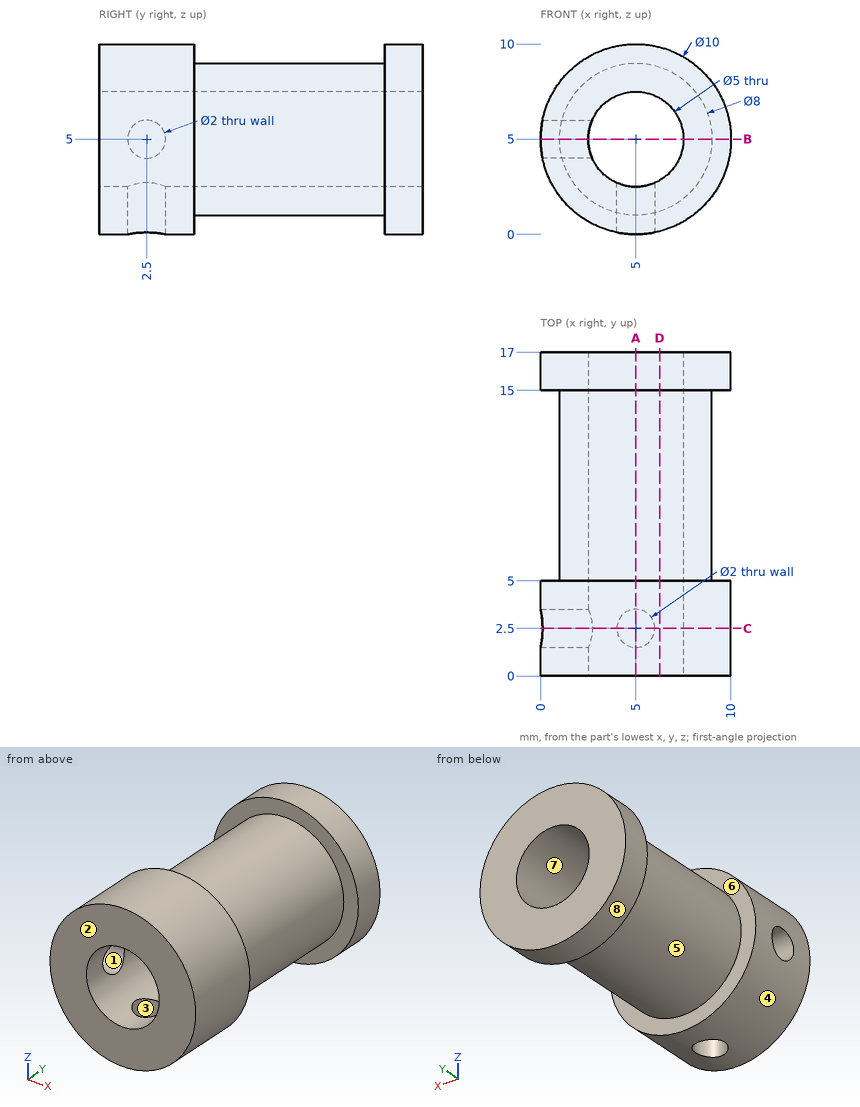
Input: dimensioned drawing with shaded views. Units: mm. Origin: part minimum x, y, z. A direction names the side the tool comes from. Coordinates: 2 decimals unless noted, no trailing zeros. Order: outer loops, then holes, each group sorted by start corner. A loop starts at its lowest first (then second) coordinate and runs counter-clockwise, first axis right, second up. Notation, with made-up numbers: (55.5, 65.5) - (112.5, 65.5) arc R15 ccw to (112.5, 80.5) - close; hole circle Ø4 at (9.25, 67.25). An arc over 180 degrees is marked (long way). Put each result on its own line as item: value.
1. Reachability of the marked faces 1, 2, 3, 4 and 5 from +Z, -Z, +X, -X, +Y, -Y: full face, straight path, thin tool, end or side. Return the list, or none.
Report:
face 1: -X
face 2: +Z, -Z, +X, -X, -Y
face 3: -Z
face 4: +Y, -Y
face 5: none
2. Cut plane A-A on x = 5. Return the cut outline in (y, z), then the cut area to 3 significant figures.
Report:
outline: (0, 0) - (1.5, 0) - (1.5, 2.5) - (0, 2.5) - close; (0, 7.5) - (17, 7.5) - (17, 10) - (15, 10) - (15, 9) - (5, 9) - (5, 10) - (0, 10) - close; (3.5, 0) - (5, 0) - (5, 1) - (15, 1) - (15, 0) - (17, 0) - (17, 2.5) - (3.5, 2.5) - close
area: 60.0 mm2
3. Draft query along Z for the marked faces 6, 7 and 8. Return one class per face: pulls with the +Z half, pulls with the -Z half, needs draft (parallel to the pull), parting line crosses it, or undercut.
Report:
face 6: needs draft
face 7: undercut
face 8: parting line crosses it
4. Cut plane B-B on z = 5. Return the cut outline in (x, y), then the cut area to 3 significant figures.
Report:
outline: (0, 0) - (2.5, 0) - (2.5, 1.5) - (0, 1.5) - close; (0, 3.5) - (2.5, 3.5) - (2.5, 17) - (0, 17) - (0, 15) - (1, 15) - (1, 5) - (0, 5) - close; (7.5, 0) - (10, 0) - (10, 5) - (9, 5) - (9, 15) - (10, 15) - (10, 17) - (7.5, 17) - close
area: 60.0 mm2
5. Contact query for flat-ended pins moving along their axis: pin 1 Ø4 at (x, y) = (6.5, 6.5) entering from +Z; pin 2 Ø3 at (y, z) = (9.5, 1.5) entering from -X; pin 3 Ø6 at (y, z) = (10.5, 8) entering from -X. Output: stop coordinate, or through.
Report:
pin 1: stops at z = 10
pin 2: stops at x = 1.54
pin 3: stops at x = 1
6. Line query: line 1 along Y through (x, z) = (6.75, 9); line 2 along Z through (x, y) = (3, 2); line 3 along Y through (x, z) = (5, 1.7). Output: solid intervals per line, ascending.
Report:
line 1: y = 0 to 5, 15 to 17
line 2: z = 0.42 to 3.5, 6.5 to 9.58
line 3: y = 0 to 1.5, 3.5 to 17
7. Cut plane C-C on y = 2.5. Return the cut outline in (x, z), then the cut area to 3 significant figures.
Report:
outline: (0.1, 4) arc R5 ccw to (4, 0.1) - (4, 2.71) arc R2.5 cw to (2.71, 4) - close; (0.1, 6) - (2.71, 6) arc R2.5 cw (long way) to (6, 2.71) - (6, 0.1) arc R5 ccw (long way) to start
area: 48.8 mm2
8. Cut plane D-D on x = 6.25. Return the cut outline in (y, z), then the cut area to 3 significant figures.
Report:
outline: (0, 0.16) - (5, 0.16) - (5, 1.2) - (15, 1.2) - (15, 0.16) - (17, 0.16) - (17, 2.83) - (0, 2.83) - close; (0, 7.17) - (17, 7.17) - (17, 9.84) - (15, 9.84) - (15, 8.8) - (5, 8.8) - (5, 9.84) - (0, 9.84) - close
area: 70.2 mm2
